Build history of the part. All positions in model axes, mm. Round coordinates to 2 decimals unless told otherwise and drop trailing zeros. Order: outer loops, then holes, each group sorted by start corner. A loop starts at its lowest first (then second) coordinate and runs counter-clockwise, first axis right, second up. Notation, with made-up numbers: M 42.25,1 L 62.25,1 A28 ccw 62.25,28 Z; hole C -8.5,32 d1. An arc over 180 degrees is marked long. One line per item, written item: value. Start each with the question number.
Item 1: Pin check, flat tips, straight feed: pin 1 (1.5 mm diameter, centred on y = 14, z = 2, fed in from -X); pin 2 (1 mm diameter, centred on x = 11, z = 0.5, fed in from -Y). Stop position of each tip, or through.
Item 2: Two-plate mould, pull along Y, no slides. Class faces 1 (the flat face through (4.4, 0.3, 4)), 2 (the cylindrical face through (0.53, 9.02, 1.97)), 3 (the cylindrical face through (20.03, -6.31, 1.97)): +Y half, -Y half, draft (parallel to the pull), parting line (faces both ways), or undercut.
Item 3: Band-saw the part on B-B, the plane y = 8. Write the cut outline in (x, z).
Item 4: Band-saw the part on D-D, the plane z = 3.3. Give the number of separate pieces and of enclosed holes in the cut face, then the cut area to 3 significant figures.
Item 5: Band-saw the part on A-A, the plane x = 0. Write the cut outline in (y, z), then the cut area to 3 significant figures.
Item 6: Probe L1, parallel to Y at x = 0, z = 2.75; L2, parallel to Y at x = -1, z = 0.7; L3, parallel to Y at x = 12, z = 2.1. List the from-to ranges inside material, lowest first.
Solid Edge part; units mm, degrees
sketch "Sketch1" plane through (0, 0, 0) normal (0, 0, 1) x (1, 0, 0)
  circle A0 centre (0, 0) radius 21
  circle A1 centre (0, 0) radius 4
  circle A2 centre (8, 0) radius 1.15
  circle A3 centre (0, 8) radius 1.15
  circle A4 centre (-8, 0) radius 1.15
  circle A5 centre (0, -8) radius 1.15
  circle A6 centre (11.3137, 11.3137) radius 1.7
  circle A7 centre (-11.3137, 11.3137) radius 1.7
  circle A8 centre (-11.3137, -11.3137) radius 1.7
  circle A9 centre (11.3137, -11.3137) radius 1.7
extrude "Protrusion1" add sketch "Sketch1" along normal blind 4
Output:
1. pin 1: stops at x = -16.29
1. pin 2: stops at y = -18.19
2. face 1: draft
2. face 2: undercut
2. face 3: parting line
3. outline: M -19.42,0 L -1.15,0 L -1.15,4 L -19.42,4 Z; M 1.15,0 L 19.42,0 L 19.42,4 L 1.15,4 Z
4. separate pieces: 1
4. enclosed holes: 9
4. area: 1,280 mm²
5. outline: M -21,0 L -9.15,0 L -9.15,4 L -21,4 Z; M -6.85,0 L -4,0 L -4,4 L -6.85,4 Z; M 4,0 L 6.85,0 L 6.85,4 L 4,4 Z; M 9.15,0 L 21,0 L 21,4 L 9.15,4 Z
5. area: 118 mm²
6. L1: y = -21 to -9.15, -6.85 to -4, 4 to 6.85, 9.15 to 21
6. L2: y = -20.98 to -8.57, -7.43 to -3.87, 3.87 to 7.43, 8.57 to 20.98
6. L3: y = -17.23 to -12.87, -9.76 to 9.76, 12.87 to 17.23
